The listing builds one solid part. Answer for the finished solid, in the listing's coordinates (mm). Face numbers are marked on the shaded views. Coordinates: 2 decimals unless noted, no trailing zeros. Order: outer loops, then holes, each group sorted by start corner. A loop starts at its lowest first (then second) coordinate and runs counter-clockwise, first axis right, second up.
from build123d import *

# Parameters (mm, degrees)
SKETCH1_W            = 24.5
SKETCH1_H            = 22.5
BOSS_EXTRUDE1_DEPTH  = 2
SKETCH2_W            = 2
SKETCH2_H            = 22.5
BOSS_EXTRUDE2_DEPTH  = 45
SKETCH4_W            = 24.5
SKETCH4_H            = 22.5
BOSS_EXTRUDE3_DEPTH  = 2
SKETCH3_R            = 0.375
CUT_EXTRUDE1_DEPTH   = 50
SKETCH5_R            = 1.75
BOSS_EXTRUDE4_DEPTH  = 1.25
BOSS_EXTRUDE4_TAPER  = 20
SKETCH6_R            = 0.75
CUT_EXTRUDE2_DEPTH   = 1.25
LPATTERN1_COUNT      = 5
LPATTERN1_PITCH      = 4
LPATTERN1_COUNT_DIR2 = 5
LPATTERN1_PITCH_DIR2 = 4


with BuildPart() as part:
    # Sketch1 → Boss-Extrude1 (new body)
    with BuildSketch(Plane(origin=(0, 0, 0), x_dir=(1, 0, 0), z_dir=(0, 1, 0))):
        Rectangle(SKETCH1_W, SKETCH1_H)
    extrude(amount=BOSS_EXTRUDE1_DEPTH)

    # Sketch2 → Boss-Extrude2 (add)
    with BuildSketch(Plane(origin=(0, 2, 0), x_dir=(1, 0, 0), z_dir=(0, 1, 0))):
        with Locations((11.25, 0)):
            Rectangle(SKETCH2_W, SKETCH2_H)
    extrude(amount=BOSS_EXTRUDE2_DEPTH)

    # Sketch4 → Boss-Extrude3 (add)
    with BuildSketch(Plane(origin=(0, 47, 0), x_dir=(1, 0, 0), z_dir=(0, 1, 0))):
        Rectangle(SKETCH4_W, SKETCH4_H)
    extrude(amount=BOSS_EXTRUDE3_DEPTH)

    # Sketch3 → Cut-Extrude1 (cut, through all)
    with BuildSketch(Plane.XZ):
        with Locations((-9, 8)):
            Circle(SKETCH3_R)
    cut_extrude1 = extrude(amount=-CUT_EXTRUDE1_DEPTH, mode=Mode.SUBTRACT)

    # Sketch5 → Boss-Extrude4 (add)
    with BuildSketch(Plane(origin=(0, 2, 0), x_dir=(1, 0, 0), z_dir=(0, 1, 0))):
        with Locations((-9, -8)):
            Circle(SKETCH5_R)
    boss_extrude4 = extrude(amount=BOSS_EXTRUDE4_DEPTH, taper=BOSS_EXTRUDE4_TAPER)

    # Sketch6 → Cut-Extrude2 (cut)
    with BuildSketch(Plane(origin=(0, 3.25, 0), x_dir=(1, 0, 0), z_dir=(0, 1, 0))):
        with Locations((-9, -8)):
            Circle(SKETCH6_R)
    cut_extrude2 = extrude(amount=-CUT_EXTRUDE2_DEPTH, mode=Mode.SUBTRACT)

    # LPattern1: Cut-Extrude1, Boss-Extrude4, Cut-Extrude2 5 × 5
    with Locations(*[(j * LPATTERN1_PITCH_DIR2, 0, -i * LPATTERN1_PITCH) for i in range(LPATTERN1_COUNT) for j in range(LPATTERN1_COUNT_DIR2) if (i, j) != (0, 0)]):
        add(cut_extrude1, mode=Mode.SUBTRACT)
        add(boss_extrude4)
        add(cut_extrude2, mode=Mode.SUBTRACT)


solid = part.part
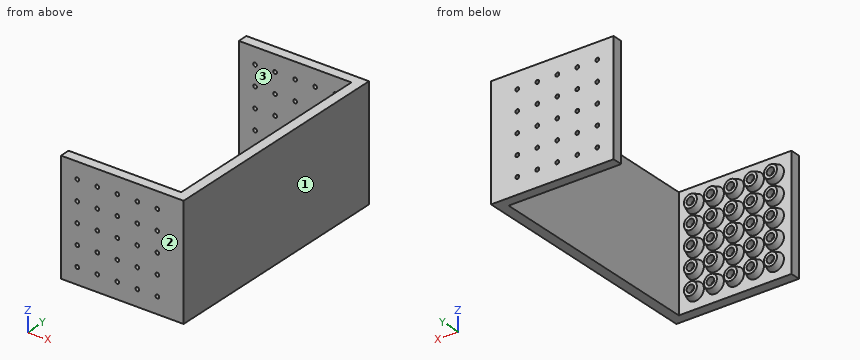
(1) The mould has two halves that part along Y. Classify the marked faces 1, 2 and 3: pulls with the +Y half, pulls with the -Y half, needs draft (parallel to the pull), parting line crosses it, or undercut.
(2) Given pin 1 Ø12 at (x, y) = (3.5, 32.5) entering from +Z; pin 2 Ø2 at (y, z) = (36.5, 2) entering from -X, each flat-ended and moving along its own axis, determine where each tip first touches the part or whether it passes through.
(3) Find the intervals of material crossed by probe 1 along Y at (x, z) = (3.75, -5); probe 2 along Y at (x, z) = (1, 8); probe 3 along Z at (x, y) = (7, 1.35) (3 decimals), in increasing order.
(4) Find section A-A on y = 20.5. Determine the outline of the cut face in (x, z).
Resolved:
1. face 1: needs draft
1. face 2: pulls with the -Y half
1. face 3: undercut
2. pin 1: passes through
2. pin 2: stops at x = 10.25
3. probe 1: y = 0 to 3.25, 47 to 49
3. probe 2: y = 0 to 2, 47 to 49
3. probe 3: z = -11.25 to -8.375, -7.625 to -4.375, -3.625 to -0.375, 0.375 to 3.625, 4.375 to 7.625, 8.375 to 11.25
4. outline: (10.25, -11.25) - (12.25, -11.25) - (12.25, 11.25) - (10.25, 11.25) - close
